Job drawing, mm, ordinate dimensions from the low corner. One solid piece. Give positions to 0.01 mm unless a question says otherwise; leave off trailing zeros. Write each loop counter-clockwise with the first axis right and the second up, starting at its lowest first coordinate (ties: lowest second). Pieces come first, ordered by that corner, then holes. Notation, with made-up numbers: (-26.75, 61) -> (16.25, 61) arc R34 cw to (16.25, 91) -> close; hole circle Ø7 at (-26.5, 56.5). An arc over 180 degrees is marked (long way). Put each result on its own line as item: value. Start each with the question number.
Item 1: Slice it at C-C, the plane z = 24. List the corners of the cut face in (x, y).
Item 2: Slice it at A-A, the plane x = 100. List the corners of the cut face in (y, z).
Item 3: Flat gauge pins, fed straight in: pin 1 Ø5 at (x, z) = (123, 14.5) entering from +Y; pin 2 Ø8 at (x, z) = (49, 12) entering from -Y; pin 3 Ø6 at (y, z) = (89.5, 10.5) entering from +X. Where does each tip first touch, or does it go through?
Item 4: Slice it at D-D, the plane y = 59. List the corners of the cut face in (x, z).
Item 5: Two-plate mould, pull along X, no slides. Class the marked faces 1, 2 and 3: pulls with the +X half, pulls with the -X half, needs draft (parallel to the pull), parting line crosses it, or undercut.
Item 6: Drill centre lines: line 1 along Y through (x, z) = (100, 11.5); line 2 along X through (y, z) = (43, 22.75); line 3 along X through (y, z) = (64, 9.5) (3 decimals). Where is each one in solid material? Low to high.
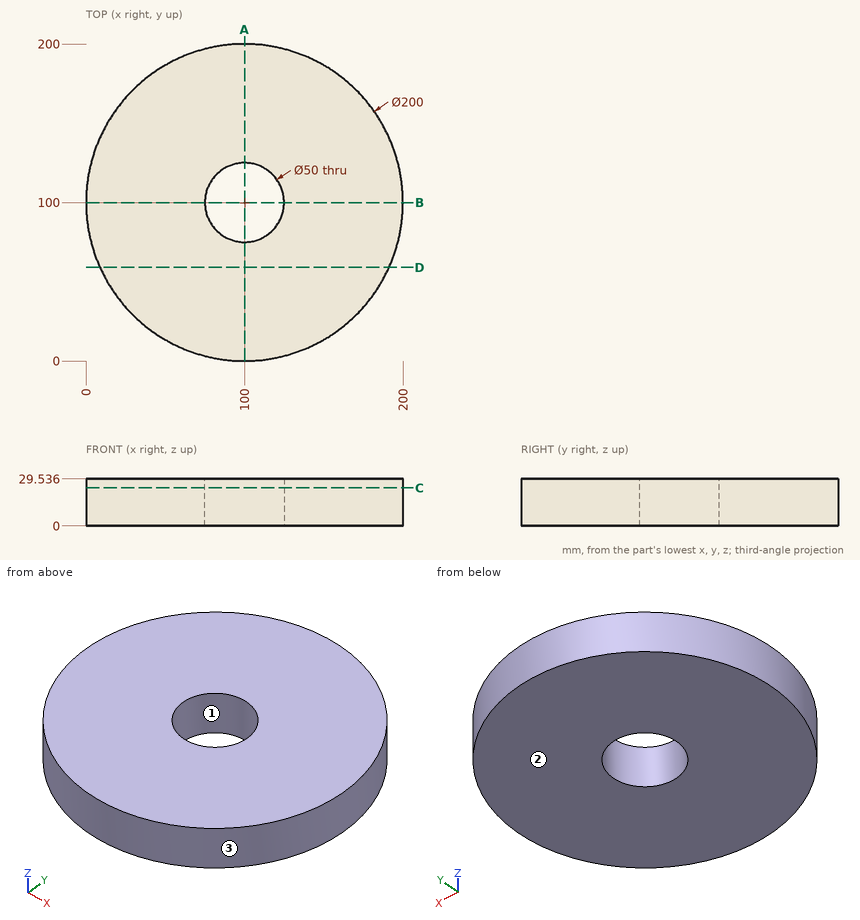
Values follow:
1. outline: circle Ø200 at (100, 100); hole circle Ø50 at (100, 100)
2. outline: (0, 0) -> (75, 0) -> (75, 29.54) -> (0, 29.54) -> close; (125, 0) -> (200, 0) -> (200, 29.54) -> (125, 29.54) -> close
3. pin 1: y = 197.88
3. pin 2: y = 11.73
3. pin 3: x = 199.72
4. outline: (8.79, 0) -> (191.21, 0) -> (191.21, 29.54) -> (8.79, 29.54) -> close
5. face 1: undercut
5. face 2: needs draft
5. face 3: parting line crosses it
6. line 1: 0 to 75, 125 to 200
6. line 2: 17.84 to 182.16
6. line 3: 6.705 to 193.295
